Here's the drawing with two shaded views (mm, measured from the low corner). I have some questions. Give positions to 0.01 mm unless a question says otherwise; leave off trailing zeros. Order: outer loops, then holes, each group sorted by start corner. A loop starts at its lowest first (then second) coordinate and runs counter-clockwise, first axis right, second up. Notation, with made-up numbers: M 60.5,9.25 L 109.5,9.25 A14 cw 109.5,29.25 Z; hole C -28.75,-6 d7. An arc over 180 degrees is marked long. Use a Markdown table: item, result. Add a question column.
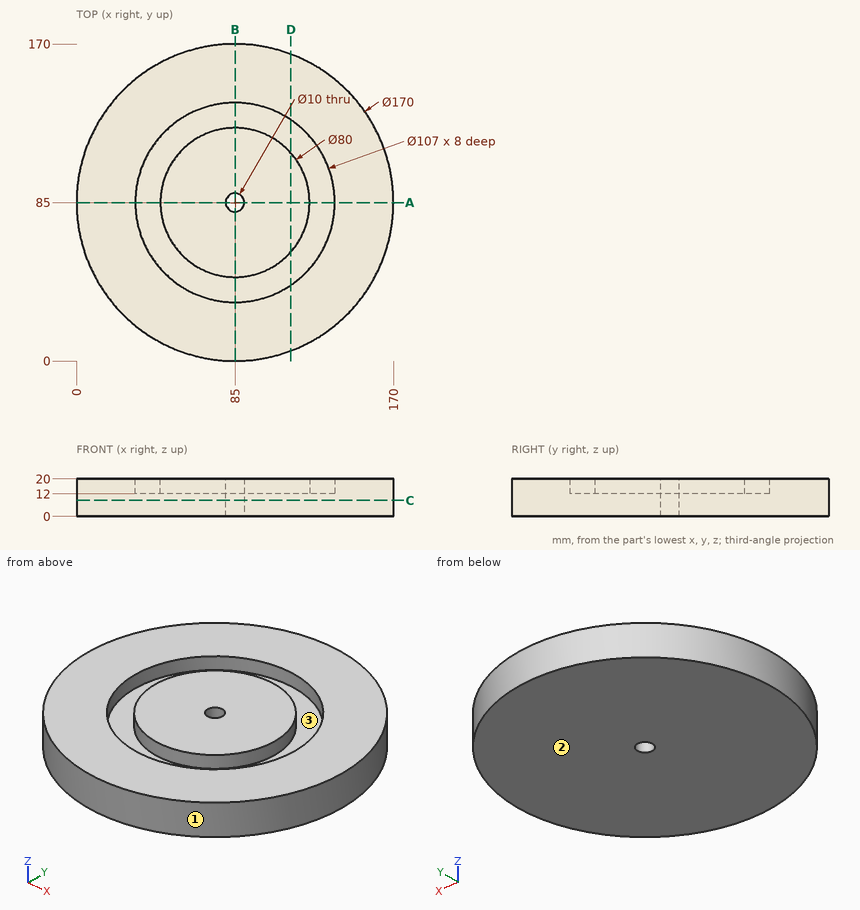
1) Suppose I cut it at A-A on y = 85. Please give me the cut outline in (x, z), and give its area (3 significant figures).
2) For pin 1 (1.5 mm diameter, centred on y = 108, z = 7.5, fed in from +X); pin 2 (1.5 mm diameter, centred on x = 17.5, z = 12.5, fed in from +Y); pin 3 (6 mm diameter, centred on x = 85, y = 85, fed in from -Z); pin 4 (2 mm diameter, centred on y = 39, z = 10.5, fed in from +X), each with a flat end and sliding along its axis, tell me the tip position at first contact or that it passes through.
3) We'd pull the mould along X, two halves only. Please class the marked faces 1, 2 and 3: pulls with the +X half, pulls with the -X half, needs draft (parallel to the pull), parting line crosses it, or undercut.
4) Suppose I cut it at D-D on x = 115. Please give me the cut outline in (y, z).
5) Please list where these lines run through material, in increasing order: line 1 (Y direction, x = 85, z = 18.25); line 2 (Y direction, x = 110, z = 13.5); line 3 (X direction, y = 76, z = 17). Write a range as from..to.
6) Suppose I cut it at C-C on z = 8.5. Please give me the cut outline in (x, y), and give its area (3 significant figures).
Values found:
| question | item | result |
|---|---|---|
| 1 | outline | M 0,0 L 80,0 L 80,20 L 45,20 L 45,12 L 31.5,12 L 31.5,20 L 0,20 Z; M 90,0 L 170,0 L 170,20 L 138.5,20 L 138.5,12 L 125,12 L 125,20 L 90,20 Z |
| 1 | area | 2,980 mm^2 |
| 2 | pin 1 | stops at x = 167.04 |
| 2 | pin 2 | stops at y = 137.63 |
| 2 | pin 3 | passes through |
| 2 | pin 4 | stops at x = 157.11 |
| 3 | face 1 | parting line crosses it |
| 3 | face 2 | needs draft |
| 3 | face 3 | undercut |
| 4 | outline | M 5.47,0 L 164.53,0 L 164.53,20 L 129.3,20 L 129.3,12 L 111.46,12 L 111.46,20 L 58.54,20 L 58.54,12 L 40.7,12 L 40.7,20 L 5.47,20 Z |
| 5 | line 1 | y = 0..31.5, 45..80, 90..125, 138.5..170 |
| 5 | line 2 | y = 3.76..37.7, 53.78..116.22, 132.3..166.24 |
| 5 | line 3 | x = 0.48..32.26, 46.03..123.97, 137.74..169.52 |
| 6 | outline | C 85,85 d170; hole C 85,85 d10 |
| 6 | area | 22,600 mm^2 |
